Autodesk Inventor part; units mm, degrees
ref_plane "YZ Plane" through (0, 0, 0) normal (1, 0, 0) x (0, 1, 0)
ref_plane "XZ Plane" through (0, 0, 0) normal (0, 1, 0) x (-1, 0, 0)
ref_plane "XY Plane" through (0, 0, 0) normal (0, 0, 1) x (1, 0, 0)
sketch "Sketch1" plane through (0, 0, 0) normal (0, 0, 1) x (1, 0, 0)
  line L0 (0, 0) -> (185, 0)
  line L1 (185, 0) -> (185, 450)
  line L2 (185, 450) -> (0, 450)
  line L3 (0, 450) -> (0, 0)
  dimension "d0" = 185
  dimension "d1" = 450
extrude "Extrusion1" add sketch "Sketch1" along normal blind 400
sketch "Sketch2" plane through (0, 0, 0) normal (-1, 0, 0) x (0, 0, 1)
  line L0 (0, 0) -> (0, 450)
  line L1 (0, 0) -> (194.069, 208.7157)
  line L2 (194.069, 208.7157) -> (0, 389.1658)
  line L3 (0, 0) -> (0, 389.1658)
  line L4 (0, 450) -> (0, 0)
  line L5 (0, 0) -> (400, 0)
  line L6 (400, 450) -> (400, 0)
  line L7 (0, 450) -> (400, 450)
  dimension "d4" = 265
  dimension "d5" = 90
  dimension "d6" = 285
extrude "Extrusion2" cut sketch "Sketch2" against normal blind 400 contours L1 L2 L0 L7 L6 L5
sketch "Sketch3" plane through (0, 208.7157, 194.069) normal (0, -0.6809437, 0.7323357) x (1, 0, 0)
  line L0 (34.9517, -115.3139) -> (34.9517, -157.3139)
  line L1 (48.9517, -171.3139) -> (58.9517, -171.3139)
  line L2 (48.9517, -101.3139) -> (54.9517, -101.3139)
  circle A0 centre (54.9517, -116.5313) radius 15.2174
  circle A1 centre (58.9517, -151.5313) radius 19.7826
  line L3 (58.9517, -131.7487) -> (54.9517, -131.7487)
  arc A2 (48.9517, -101.3139) -> (34.9517, -115.3139) centre (48.9517, -115.3139) ccw
  arc A3 (34.9517, -157.3139) -> (48.9517, -171.3139) centre (48.9517, -157.3139) ccw
  circle A4 centre (128.9517, -136.3139) radius 35
  circle A5 centre (128.9517, -136.3139) radius 17.5
  circle A6 centre (142.9517, -114.1089) radius 8.75
  circle A7 centre (142.9517, -158.5189) radius 8.75
  point P0 (0, -285)
  point P1 (0, 0)
  point P2 (34.9517, -101.3139)
  point P3 (34.9517, -171.3139)
  point P4 (34.9517, -136.3139)
  point P5 (135.9261, 202.4385)
  point P6 (135.9261, 232.0451)
  point P7 (145.2595, 246.8485)
  point P8 (145.2595, 187.6351)
  point P9 (52.5928, 252.2418)
  point P10 (56.5928, 182.2418)
  point P11 (138.285, -151.1172)
  point P12 (138.285, -121.5105)
  point P13 (147.6184, -106.7072)
  point P14 (147.6184, -165.9206)
  point P15 (58.9517, -171.3139)
  dimension "d12" = 30.4348
  dimension "d13" = 39.5652
  dimension "d9" = 70
  dimension "d10" = 24
  dimension "d11" = 20
  dimension "d14" = 15.2174
  dimension "d15" = 19.7826
  dimension "d16" = 14
  dimension "d17" = 70
  dimension "d18" = 35
  dimension "d19" = 17.5
  dimension "d20" = 17.5
  dimension "d21" = 14
  dimension "d22" = 70
extrude "Extrusion3" cut sketch "Sketch3" against normal blind 10 contours A2 L2 A0 L3 A1 L1 A3 L0 | A0 | A1 | A6 A5 A7 A4 | A6 | A7 picked at (128.1694, -161.6024)
equation "\"d12\" = 0.434783 * d9"
equation "\"d13\" = d9 - d12"
equation "\"d16\" = 0.2 * d9"
equation "\"d17\" = d9"
equation "\"d18\" = 0.5 * d17"
equation "\"d19\" = -0.5 * d18 + 0.5 * d17"
equation "\"d20\" = d19"
equation "\"d21\" = 0.2 * d17"
properties part number "Triangle_V3"
Geometry check sheet. Reference: the model listing, model coordinates, mm. A direction names the side the tool comes from. Give positions to 0.01 mm unless a question says otherwise; leave off trailing zeros. Loops run counter-clockwise (first coordinate to the right, second up) from the corner with the lowest first, then second, coordinate; pieces in that order, holes last. Notation, with made-up numbers: M 66,16.25 L 80,16.25 A24 ccw 80,34.25 Z; hole C 89.5,60 d6. An arc over 180 degrees is marked long. Write item = value, one per line. Start each with the question number.
1. Section check B-B, the plane z = 150. Enter the section's corners in (x, y), plus the area to 3 significant figures.
2. Section check C-C, the plane y = 193.5. Enter the section's corners in (x, z), plus the area to 3 significant figures.
3. Tool access check on faces 5 (the face through (39.16, 134.95, 118.75)), 6 (the face through (78.73, 100.78, 86.98)), 7 (the face through (38.94, 89.7, 76.67)). Record the directions out of +Z, -Z, +X, -X, +Y, -Y that give a thin tool (end or side, any length) a straight path to the whole face; none if there is none.
4. Section check D-D, the plane x = 105. Enter the section's corners in (y, z), plus the area to 3 significant figures.
5. Section check A-A, the plane x = 143. Enter the section's corners in (y, z).
6. Draft check along X on faces 1 (the face through (91.2, 297.68, 98.39)), 2 (the face through (109.59, 116.06, 94.26)), 3 (the face through (34.952, 112, 98)), 4 (the face through (0, 197, 74)). Enter one of: +X half, -X half, draft (parallel to the pull), parting line (faces both ways), or undercut.
7. Thickness scan on probe 1 along Z at (x, y) = (96.5, 285.5); probe 2 along Z at (x, y) = (48.5, 174.5); probe 3 along Y at (x, z) = (105, 60.5). Record the ranges inside material, lowest first.
8. Go/stop test with flat-tipped pins: P1, Ø8, axis at x = 103, z = 163.5, coming from the +Y side; P2, Ø2, axis at x = 138.5, y = 232.5, coming from the -Z side; P3, Ø8, axis at x = 25, z = 36.5, coming from the -Y side; P4, Ø2, axis at x = 46.5, y = 76, coming from the +Z side. Record where each tip stops, or that it passes through.
Values follow:
q1.outline = M 0,161.32 L 185,161.32 L 185,249.69 L 0,249.69 Z
q1.area = 16,300 mm^2
q2.outline = M 0,0 L 185,0 L 185,179.92 L 0,179.92 Z
q2.area = 33,300 mm^2
q3.face_5 = -Y
q3.face_6 = none
q3.face_7 = +Z
q4.outline = M 0,0 L 389.17,0 L 208.72,194.07 L 127.58,118.63 L 134.39,111.3 L 97.01,76.54 L 90.2,83.87 Z
q4.area = 37,300 mm^2
q5.outline = M 0,0 L 389.17,0 L 208.72,194.07 L 132.36,123.08 L 139.18,115.75 L 125.55,103.08 L 118.74,110.41 L 99.03,92.08 L 105.85,84.76 L 92.22,72.09 L 85.41,79.42 Z
q6.face_1 = draft
q6.face_2 = undercut
q6.face_3 = undercut
q6.face_4 = -X half
q7.probe_1 = 0 to 111.49
q7.probe_2 = 0 to 162.25
q7.probe_3 = 65.07 to 332.91
q8.P1 = 240.86
q8.P2 = 0
q8.P3 = 34.95
q8.P4 = 71.6
